Here's how the part is built. I have some questions about the finished solid (model axes, mm). Coordinates: 2 decimals unless noted, no trailing zeros. Write each loop counter-clockwise with the first axis right and the second up, starting at its lowest first coordinate (ties: lowest second). Pieces come first, ordered by that corner, then holes. Notation, with made-up numbers: (-22.75, 6.5) -> (28.25, 6.5) arc R22 cw to (28.25, 37.5) -> close; hole circle Ø9 at (47.5, 5). An arc over 180 degrees is marked (long way). Put each result on its own line as item: value. Start each with the question number.
Item 1: I want a section at C-C, the plane y = -11.5. List the corners of the cut face in (x, z) for me.
Item 2: I want a section at B-B, the plane y = 31.75. List the corners of the cut face in (x, z) for me, then the cut area to 3 significant figures.
Item 3: I want a section at A-A, the plane y = -31.75. List the corners of the cut face in (x, z) for me.
Item 4: I want a section at D-D, the plane x = 152.4. List the corners of the cut face in (y, z) for me.
Item 5: For pin 1 (5 mm diameter, centred on y = 33, z = 8.5, fed in from +X); pin 2 (3 mm diameter, centred on y = 31, z = 10.5, fed in from -X); pin 3 (12 mm diameter, centred on x = -162, y = 25.5, fed in from -Z), each with a flat end and sliding along its axis, tell me the tip position at first contact or that it passes through.
Item 6: I need wall thicknesses on line 1 (X direction, y = -3.5, z = 1.25); line 2 (Z direction, x = -239, y = -31). Which ranges of each line are inside material? Lowest first, please. Write a range as [from, to].
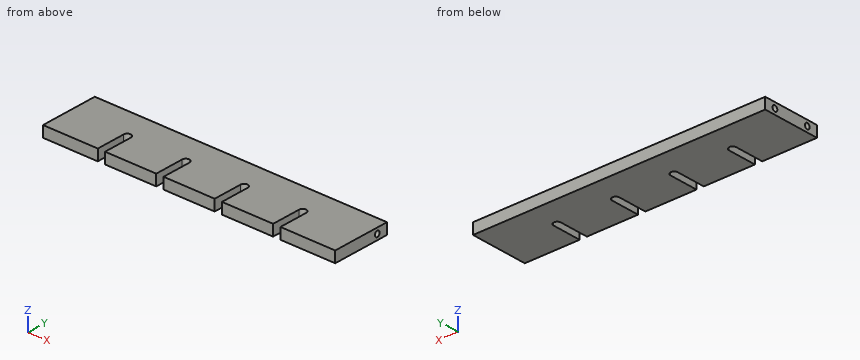
from build123d import *

# Parameters (mm, degrees)
F1_DEPTH = 19.05
F2_R     = 4.7625
F3_DEPTH = 25.4
F4_R     = 4.7625
F5_DEPTH = 25.4


with BuildPart() as f1:
    # F0 (on Top) → F1 (new body)
    with BuildSketch(Plane.XY):
        with BuildLine():
            Line((254, -50.8), (254, 50.8))
            Line((254, 50.8), (-254, 50.8))
            Line((-254, 50.8), (-254, -50.8))
            Line((-254, -50.8), (-158.75, -50.8))
            Line((-158.75, -50.8), (-158.75, 0))
            ThreePointArc((-158.75, 0), (-152.4, 6.35), (-146.05, 0))
            Line((-146.05, 0), (-146.05, -50.8))
            Line((-146.05, -50.8), (-57.15, -50.8))
            Line((-57.15, -50.8), (-57.15, 0))
            ThreePointArc((-57.15, 0), (-50.8, 6.35), (-44.45, 0))
            Line((-44.45, 0), (-44.45, -50.8))
            Line((-44.45, -50.8), (44.45, -50.8))
            Line((44.45, -50.8), (44.45, 0))
            ThreePointArc((44.45, 0), (50.8, 6.35), (57.15, 0))
            Line((57.15, 0), (57.15, -50.8))
            Line((57.15, -50.8), (146.05, -50.8))
            Line((146.05, -50.8), (146.05, 0))
            ThreePointArc((146.05, 0), (152.4, 6.35), (158.75, 0))
            Line((158.75, 0), (158.75, -50.8))
            Line((158.75, -50.8), (254, -50.8))
        make_face()
    extrude(amount=F1_DEPTH)

    # F2 (on face) → F3 (cut)
    with BuildSketch(Plane.YZ.offset(254)):
        with Locations((31.75, 9.525)):
            Circle(F2_R)
    extrude(amount=-F3_DEPTH, mode=Mode.SUBTRACT)

    # F4 (on face) → F5 (cut)
    with BuildSketch(Plane(origin=(-254, 0, 0), x_dir=(0, -1, 0), z_dir=(-1, 0, 0))):
        with Locations((-31.75, 9.525)):
            Circle(F4_R)
        with Locations((31.75, 9.525)):
            Circle(F4_R)
    extrude(amount=-F5_DEPTH, mode=Mode.SUBTRACT)


solid = f1.part
Calculated:
1. outline: (-254, 0) -> (-158.75, 0) -> (-158.75, 19.05) -> (-254, 19.05) -> close; (-146.05, 0) -> (-57.15, 0) -> (-57.15, 19.05) -> (-146.05, 19.05) -> close; (-44.45, 0) -> (44.45, 0) -> (44.45, 19.05) -> (-44.45, 19.05) -> close; (57.15, 0) -> (146.05, 0) -> (146.05, 19.05) -> (57.15, 19.05) -> close; (158.75, 0) -> (254, 0) -> (254, 19.05) -> (158.75, 19.05) -> close
2. outline: (-254, 0) -> (254, 0) -> (254, 4.76) -> (228.6, 4.76) -> (228.6, 14.29) -> (254, 14.29) -> (254, 19.05) -> (-254, 19.05) -> (-254, 14.29) -> (-228.6, 14.29) -> (-228.6, 4.76) -> (-254, 4.76) -> close
2. area: 9,190 mm2
3. outline: (-254, 0) -> (-158.75, 0) -> (-158.75, 19.05) -> (-254, 19.05) -> (-254, 14.29) -> (-228.6, 14.29) -> (-228.6, 4.76) -> (-254, 4.76) -> close; (-146.05, 0) -> (-57.15, 0) -> (-57.15, 19.05) -> (-146.05, 19.05) -> close; (-44.45, 0) -> (44.45, 0) -> (44.45, 19.05) -> (-44.45, 19.05) -> close; (57.15, 0) -> (146.05, 0) -> (146.05, 19.05) -> (57.15, 19.05) -> close; (158.75, 0) -> (254, 0) -> (254, 19.05) -> (158.75, 19.05) -> close
4. outline: (6.35, 0) -> (50.8, 0) -> (50.8, 19.05) -> (6.35, 19.05) -> close
5. pin 1: stops at x = 228.6
5. pin 2: stops at x = -228.6
5. pin 3: stops at z = 0
6. line 1: x = [-254, -158.75], [-146.05, -57.15], [-44.45, 44.45], [57.15, 146.05], [158.75, 254]
6. line 2: z = [0, 4.82], [14.23, 19.05]
